Job drawing, mm, ordinate dimensions from the low corner. One solid piece. Give positions to 0.01 mm unless a question says otherwise; leave off trailing zeros. Order: outer loops, then holes, each group sorted by start corner. A loop starts at its lowest first (then second) coordinate and runs counter-clockwise, first axis right, second up. Notation, with made-up numbers: (82, 53) -> (132, 53) arc R32 ccw to (132, 89) -> close; hole circle Ø4 at (-24.75, 83). An arc over 180 degrees is marked (long way). Use CSV: the item, a comma, the result in double quotes. Start each with the question number.
1. Cut at A-A on y = 51. List the corners of the cut face in (x, z).
2. Pull direction Z, two halves, no side cores. Call the marked faces 1 and 2: released by +Z, released by -Z, zero draft, split by the parting line, or undercut.
3. Wall check: line 1 (X direction, y = 44.5, z = 4.75); line 2 (Z direction, x = 0.5, y = 29.5). Give the ranges that are in metal, low to high. Write a range as from..to.
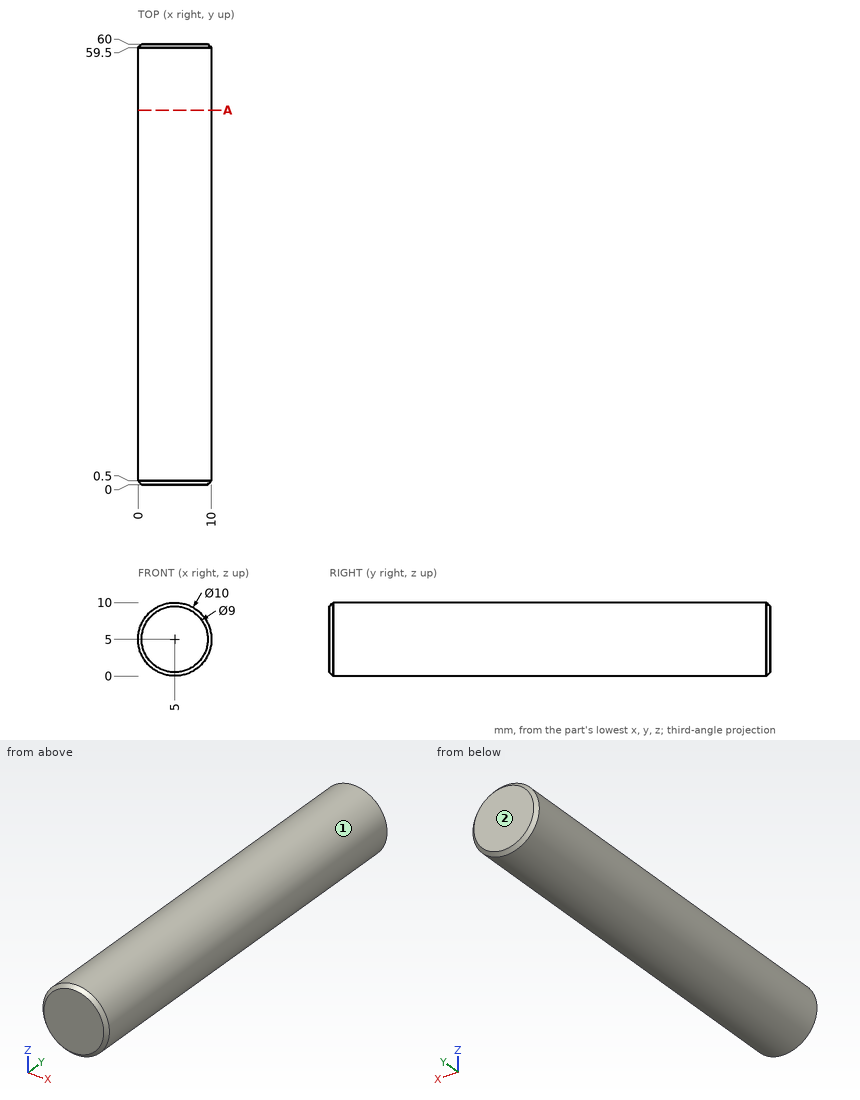
Verdict:
1,outline,"circle Ø10 at (5, 5)"
2,face 1,"split by the parting line"
2,face 2,"zero draft"
3,line 1,"0.01..9.99"
3,line 2,"2.82..7.18"
